Build history of the part. All positions in model axes, mm. Face numbers are marked on the shaded views. A direction names the side the tool comes from. Round coordinates to 2 decimals unless told otherwise and drop trailing zeros. Write each loop counter-clockwise with the first axis right and the second up, starting at its lowest first coordinate (ties: lowest second). Pieces come first, ordered by that corner, then holes. Notation, with made-up numbers: (83, 37) -> (125, 37) arc R21 ccw to (125, 64) -> close; hole circle Ø1 at (3.25, -2.5). An arc over 180 degrees is marked (long way). Answer as CSV lines item,"result".
from build123d import *

# Parameters (mm, degrees)
SKETCH1_W           = 50.8
SKETCH1_H           = 38.1
BOSS_EXTRUDE1_DEPTH = 50.8
SKETCH2_W           = 38.1
SKETCH2_H           = 38.1
CUT_EXTRUDE1_DEPTH  = 38.1
SKETCH3_R           = 5.588
CUT_EXTRUDE2_DEPTH  = 4.064
SKETCH4_R           = 3.302
CUT_EXTRUDE3_DEPTH  = 8.636
SKETCH5_R           = 5.588
CUT_EXTRUDE4_DEPTH  = 4.064
SKETCH6_R           = 3.302
CUT_EXTRUDE5_DEPTH  = 8.636
FILLET1_R           = 38.1


with BuildPart() as part:
    # Sketch1 → Boss-Extrude1 (new body)
    with BuildSketch(Plane(origin=(0, 0, 0), x_dir=(1, 0, 0), z_dir=(0, 1, 0))):
        with Locations((25.4, -19.05)):
            Rectangle(SKETCH1_W, SKETCH1_H)
    extrude(amount=BOSS_EXTRUDE1_DEPTH)

    # Sketch2 → Cut-Extrude1 (cut)
    with BuildSketch(Plane.XY.offset(38.1)):
        with Locations((31.75, 31.75)):
            Rectangle(SKETCH2_W, SKETCH2_H)
    extrude(amount=-CUT_EXTRUDE1_DEPTH, mode=Mode.SUBTRACT)

    # Sketch3 → Cut-Extrude2 (cut)
    with BuildSketch(Plane(origin=(0, 12.7, 0), x_dir=(1, 0, 0), z_dir=(0, 1, 0))):
        with Locations(Location((31.75, -19.05, 0), (0, 0, 270))):
            Circle(SKETCH3_R)
    extrude(amount=-CUT_EXTRUDE2_DEPTH, mode=Mode.SUBTRACT)

    # Sketch4 → Cut-Extrude3 (cut)
    with BuildSketch(Plane(origin=(0, 8.636, 0), x_dir=(1, 0, 0), z_dir=(0, 1, 0))):
        with Locations(Location((31.75, -19.05, 0), (0, 0, 270))):
            Circle(SKETCH4_R)
    extrude(amount=-CUT_EXTRUDE3_DEPTH, mode=Mode.SUBTRACT)

    # Sketch5 → Cut-Extrude4 (cut)
    with BuildSketch(Plane(origin=(12.7, 0, 0), x_dir=(0, 0, -1), z_dir=(1, 0, 0))):
        with Locations(Location((-19.05, 31.75, 0), (0, 0, 90))):
            Circle(SKETCH5_R)
    extrude(amount=-CUT_EXTRUDE4_DEPTH, mode=Mode.SUBTRACT)

    # Sketch6 → Cut-Extrude5 (cut)
    with BuildSketch(Plane(origin=(8.636, 0, 0), x_dir=(0, 0, -1), z_dir=(1, 0, 0))):
        with Locations(Location((-19.05, 31.75, 0), (0, 0, 90))):
            Circle(SKETCH6_R)
    extrude(amount=-CUT_EXTRUDE5_DEPTH, mode=Mode.SUBTRACT)

    # Fillet1
    # the kernel refuses this fillet: 38.1 mm, written as the material it adds along each edge
    with BuildSketch(Plane(origin=(12.7, 12.7, 38.1), x_dir=(0, 1, 0), z_dir=(0, 0, -1))) as fillet1_piece_1_section:
        with BuildLine():
            CenterArc((FILLET1_R, FILLET1_R), FILLET1_R, 180, 90)
            Line((0, FILLET1_R), (0, 0))
            Line((0, 0), (FILLET1_R, 0))
        make_face()
    fillet1_piece_1 = extrude(amount=38.1, mode=Mode.PRIVATE)
    fillet1_piece_1 = fillet1_piece_1 - Plane(origin=(21.164766811, 31.75, 19.05), x_dir=(0, 1, 0), z_dir=(1, 0, 0)) * Cylinder(5.588, 229, mode=Mode.PRIVATE)
    fillet1_piece_1 = fillet1_piece_1 - Plane(origin=(31.75, 21.164747652, 19.05), x_dir=(0, 0, 1), z_dir=(0, 1, 0)) * Cylinder(5.588, 229, mode=Mode.PRIVATE)
    add(fillet1_piece_1)

    # Chamfer1
    # the kernel refuses this chamfer: 1.27 mm, written as the material it takes off along each edge
    with BuildSketch(Plane(origin=(50.8, 12.7, 41.316229993), x_dir=(-0.9990092495059921, 0.04450302687991344, 0), z_dir=(0, 0, -1))) as chamfer1_piece_1:
        with BuildLine():
            Line((1.265623079, 0), (-0.09253308, -1.283159884))
            Line((-0.09253308, -1.283159884), (-0.117907915, -1.282029507))
            ThreePointArc((-0.117907915, -1.282029507), (-0.053990428, -0.641235865), (-0.025374835, 0.001130377))
            Line((-0.025374835, 0.001130377), (0.001130377, 0.025374835))
            ThreePointArc((0.001130377, 0.025374835), (0.632880934, 0.002485367), (1.265934324, 0.025398093))
            Line((1.265934324, 0.025398093), (1.265623079, 0))
        make_face()
    extrude(amount=44.532459986, mode=Mode.SUBTRACT)
    with BuildSketch(Plane(origin=(12.7, 50.8, 41.316229993), x_dir=(0.04450302687991419, -0.9990092495059921, 0), z_dir=(0, 0, -1))) as chamfer1_piece_2:
        with BuildLine():
            Line((1.265623079, 0), (-0.09253308, 1.283159884))
            Line((-0.09253308, 1.283159884), (-0.117907915, 1.282029507))
            ThreePointArc((-0.117907915, 1.282029507), (-0.053990428, 0.641235865), (-0.025374835, -0.001130377))
            Line((-0.025374835, -0.001130377), (0.001130377, -0.025374835))
            ThreePointArc((0.001130377, -0.025374835), (0.632880934, -0.002485367), (1.265934324, -0.025398093))
            Line((1.265934324, -0.025398093), (1.265623079, 0))
        make_face()
    extrude(amount=44.532459986, mode=Mode.SUBTRACT)
    with BuildSketch(Plane(origin=(50.8, 50.8, 38.1), x_dir=(0.08565212644692491, -0.9963251041879453, 0), z_dir=(0.9963251041879453, 0.08565212644692491, 0))) as chamfer1_piece_3:
        with BuildLine():
            Line((38.064078976, 1.305921024), (39.405921024, -0.035921024))
            Line((39.405921024, -0.035921024), (39.405921024, -0.061321024))
            ThreePointArc((39.405921024, -0.061321024), (38.752960512, -0.0254), (38.1, -0.0254))
            Line((38.1, -0.0254), (38.0746, 0))
            ThreePointArc((38.0746, 0), (38.0746, 0.652960512), (38.038678976, 1.305921024))
            Line((38.038678976, 1.305921024), (38.064078976, 1.305921024))
        make_face()
    revolve(axis=Axis((50.8, 50.8, 38.1), (0, 0, -1)), revolution_arc=99.827051452, mode=Mode.SUBTRACT)
    with BuildSketch(Plane(origin=(50.8, 50.8, 0), x_dir=(0.08565212644692491, -0.9963251041879453, 0), z_dir=(0.9963251041879453, 0.08565212644692491, 0))) as chamfer1_piece_4:
        with BuildLine():
            Line((38.064078976, -1.305921024), (39.405921024, 0.035921024))
            Line((39.405921024, 0.035921024), (39.405921024, 0.061321024))
            ThreePointArc((39.405921024, 0.061321024), (38.752960512, 0.0254), (38.1, 0.0254))
            Line((38.1, 0.0254), (38.0746, 0))
            ThreePointArc((38.0746, 0), (38.0746, -0.652960512), (38.038678976, -1.305921024))
            Line((38.038678976, -1.305921024), (38.064078976, -1.305921024))
        make_face()
    revolve(axis=Axis((50.8, 50.8, 0), (0, 0, -1)), revolution_arc=99.827051452, mode=Mode.SUBTRACT)


solid = part.part
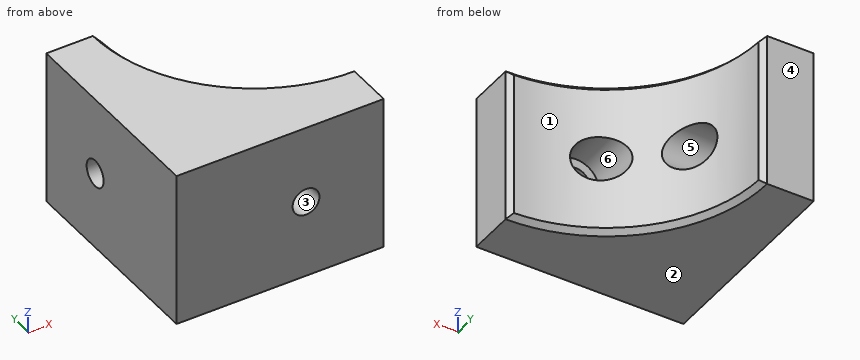
1. Drop flat-ended pins along their axis: pin 1 Ø14.5 at (x, z) = (31.75, 19.05) entering from +Y; pin 2 Ø5.5 at (x, z) = (31, 16.5) entering from +Y; pin 3 Ø6 at (y, z) = (20, 27.5) entering from +X. Give the stop position or say it passes through.
Results found:
pin 1,"stops at y = 23.23"
pin 2,"stops at y = 8.64"
pin 3,"stops at x = 33.22"
2. Cut at C-C, the plane z = 19.05. Write the cut outline in (x, y), then the cut area to 3 significant figures.
Results found:
outline,"(0, 0) -> (28.45, 0) -> (28.45, 8.64) -> (26.16, 8.64) -> (26.16, 21.74) arc R38.1 cw to (21.74, 26.16) -> (8.64, 26.16) -> (8.64, 28.45) -> (0, 28.45) -> close; (0, 35.05) -> (8.64, 35.05) -> (8.64, 37.34) -> (15.16, 37.34) arc R38.1 cw to (12.72, 49.57) -> (11.45, 50.8) -> (0, 50.8) -> close; (35.05, 0) -> (50.8, 0) -> (50.8, 11.45) -> (49.57, 12.72) arc R38.1 cw to (37.34, 15.16) -> (37.34, 8.64) -> (35.05, 8.64) -> close"
area,"1,120 mm2"
3. Probe line 1 along X through (y, z) = (6, 19.05); line 2 along Z through (x, y) = (12.25, 31.75); line 3 along Z through (x, y) = (4, 31.75). List the from-to ranges inside material, lowest first.
Results found:
line 1,"x = 0 to 28.45, 35.05 to 50.8"
line 2,"z = 0 to 13.46, 24.64 to 38.1"
line 3,"z = 0 to 15.75, 22.35 to 38.1"
4. Cut at B-B, the plane y = 9.5. Write the cut outline in (x, z), then the cut area to 3 significant figures.
Results found:
outline,"(0, 0) -> (50.8, 0) -> (50.8, 38.1) -> (0, 38.1) -> close; hole circle Ø11.18 at (31.75, 19.05)"
area,"1,840 mm2"
5. Which spindle directions (+Z, -Z, +X, -X, +Y, -Y) get a long thin tool onto all of the face, cutting with end or side? Do the marked faces 4, 5 and 6. Say none if no direction does.
Results found:
face 4,"+Z, -Z, +X, -X, +Y"
face 5,"+X"
face 6,"+Y"
6. Mould opens along X. For the marked faces 1, 2 and 3 say: +X half, -X half, draft (parallel to the pull), parting line (faces both ways), or undercut.
Results found:
face 1,"+X half"
face 2,"draft"
face 3,"undercut"
7. Cut at A-A, the plane z = 25.5. Write the cut outline in (x, y), then the cut area to 3 significant figures.
Results found:
outline,"(0, 0) -> (50.8, 0) -> (50.8, 11.45) -> (49.57, 12.72) arc R38.1 cw to (12.72, 49.57) -> (11.45, 50.8) -> (0, 50.8) -> close"
area,"1,440 mm2"
